from build123d import *

# Parameters (mm, degrees)
SKETCH_1_R          = 25.5
SKETCH_1_R_2        = 15
EXTRUDE_1_DEPTH     = 2
SKETCH_2_R          = 25.5
SKETCH_2_R_2        = 21.5
EXTRUDE_2_DEPTH     = 2
SKETCH_3_R          = 25.5
SKETCH_3_R_2        = 23.5
EXTRUDE_3_DEPTH     = 7
SKETCH_4_W          = 51
SKETCH_4_H          = 80
SKETCH_4_R          = 23.5
EXTRUDE_4_DEPTH     = 8
FILLET_1_R          = 20
SKETCH_5_W          = 51
SKETCH_5_H          = 5
EXTRUDE_5_DEPTH     = 19.7
SKETCH_6_W          = 40
SKETCH_6_H          = 70
EXTRUDE_6_DEPTH     = 3
CUT_EXTRUDE_1_REACH = 65.975
SKETCH_7_R          = 1.25
SKETCH_8_R          = 75
EXTRUDE_7_DEPTH     = 5
SKETCH_9_R          = 22.5
CUT_EXTRUDE_2_DEPTH = 2
CUT_EXTRUDE_3_REACH = 142.425
SKETCH_10_R         = 1.75


with BuildPart() as part:
    # 스케치1 → 보스-돌출1 (new body)
    with BuildSketch(Plane.XY):
        Circle(SKETCH_1_R)
        Circle(SKETCH_1_R_2, mode=Mode.SUBTRACT)
    extrude(amount=EXTRUDE_1_DEPTH)

    # 스케치2 → 보스-돌출2 (add)
    with BuildSketch(Plane.XY.offset(2)):
        Circle(SKETCH_2_R)
        Circle(SKETCH_2_R_2, mode=Mode.SUBTRACT)
    extrude(amount=EXTRUDE_2_DEPTH)

    # 스케치3 → 보스-돌출3 (add)
    with BuildSketch(Plane.XY.offset(4)):
        Circle(SKETCH_3_R)
        Circle(SKETCH_3_R_2, mode=Mode.SUBTRACT)
    extrude(amount=EXTRUDE_3_DEPTH)

    # 스케치4 → 보스-돌출4 (add)
    with BuildSketch(Plane(origin=(0, 0, 0), x_dir=(-1, 0, 0), z_dir=(0, 0, -1))):
        with Locations((0, -10)):
            Rectangle(SKETCH_4_W, SKETCH_4_H)
        with Locations(Location((0, 0, 0), (0, 0, 180))):
            Circle(SKETCH_4_R, mode=Mode.SUBTRACT)
    extrude(amount=-EXTRUDE_4_DEPTH)

    # 필렛1
    fillet_1_edges = [part.edges().sort_by_distance(p)[0] for p in [
        (-25.5, 30, 4),
        (25.5, 30, 4),
    ]]
    fillet(fillet_1_edges, radius=FILLET_1_R)

    # 스케치5 → 보스-돌출5 (add)
    with BuildSketch(Plane(origin=(0, 0, 0), x_dir=(-1, 0, 0), z_dir=(0, 0, -1))):
        Polygon((-20, 20), (-10, 20), (-10, 17), (-17, 17), (-17, 10), (-20, 10), align=None)
        Polygon((20, 20), (10, 20), (10, 17), (17, 17), (17, 10), (20, 10), align=None)
        with Locations((0, -47.5)):
            Rectangle(SKETCH_5_W, SKETCH_5_H)
    extrude(amount=EXTRUDE_5_DEPTH)

    # 스케치6 → 보스-돌출6 (add)
    with BuildSketch(Plane(origin=(0, 0, -19.7), x_dir=(-1, 0, 0), z_dir=(0, 0, -1))):
        with Locations((0, -15)):
            Rectangle(SKETCH_6_W, SKETCH_6_H)
    extrude(amount=-EXTRUDE_6_DEPTH)

    # 스케치7 → 컷-돌출1 (cut, up to next)
    with BuildSketch(Plane(origin=(0, 0, -19.7), x_dir=(-1, 0, 0), z_dir=(0, 0, -1)), mode=Mode.PRIVATE) as cut_extrude_1_sk1:
        with Locations((-5, 13.85)):
            Circle(SKETCH_7_R)
    cut_extrude_1_tool1 = extrude(cut_extrude_1_sk1.sketch, amount=-CUT_EXTRUDE_1_REACH, mode=Mode.PRIVATE) & part.part
    # 스케치7 → 컷-돌출1 (cut, up to next)
    with BuildSketch(Plane(origin=(0, 0, -19.7), x_dir=(-1, 0, 0), z_dir=(0, 0, -1)), mode=Mode.PRIVATE) as cut_extrude_1_sk2:
        with Locations((5, 13.85)):
            Circle(SKETCH_7_R)
    cut_extrude_1_tool2 = extrude(cut_extrude_1_sk2.sketch, amount=-CUT_EXTRUDE_1_REACH, mode=Mode.PRIVATE) & part.part
    # 스케치7 → 컷-돌출1 (cut, up to next)
    with BuildSketch(Plane(origin=(0, 0, -19.7), x_dir=(-1, 0, 0), z_dir=(0, 0, -1)), mode=Mode.PRIVATE) as cut_extrude_1_sk3:
        with Locations((5, -34.75)):
            Circle(SKETCH_7_R)
    cut_extrude_1_tool3 = extrude(cut_extrude_1_sk3.sketch, amount=-CUT_EXTRUDE_1_REACH, mode=Mode.PRIVATE) & part.part
    # 스케치7 → 컷-돌출1 (cut, up to next)
    with BuildSketch(Plane(origin=(0, 0, -19.7), x_dir=(-1, 0, 0), z_dir=(0, 0, -1)), mode=Mode.PRIVATE) as cut_extrude_1_sk4:
        with Locations((-5, -34.75)):
            Circle(SKETCH_7_R)
    cut_extrude_1_tool4 = extrude(cut_extrude_1_sk4.sketch, amount=-CUT_EXTRUDE_1_REACH, mode=Mode.PRIVATE) & part.part
    # 스케치7 → 컷-돌출1 (cut, up to next)
    with BuildSketch(Plane(origin=(0, 0, -19.7), x_dir=(-1, 0, 0), z_dir=(0, 0, -1)), mode=Mode.PRIVATE) as cut_extrude_1_sk5:
        Polygon((-11, -31.5), (-1, -31.5), (-1, -38), (1, -38), (1, -31.5), (11, -31.5), (11, 10.5), (1, 10.5), (1, 17), (-1, 17), (-1, 10.5), (-11, 10.5), align=None)
    cut_extrude_1_tool5 = extrude(cut_extrude_1_sk5.sketch, amount=-CUT_EXTRUDE_1_REACH, mode=Mode.PRIVATE) & part.part
    add(cut_extrude_1_tool1.solids().sort_by_distance((5, 13.85, -19.7))[0], mode=Mode.SUBTRACT)
    add(cut_extrude_1_tool2.solids().sort_by_distance((-5, 13.85, -19.7))[0], mode=Mode.SUBTRACT)
    add(cut_extrude_1_tool3.solids().sort_by_distance((-5, -34.75, -19.7))[0], mode=Mode.SUBTRACT)
    add(cut_extrude_1_tool4.solids().sort_by_distance((5, -34.75, -19.7))[0], mode=Mode.SUBTRACT)
    add(cut_extrude_1_tool5.solids().sort_by_distance((0, -10.5, -19.7))[0], mode=Mode.SUBTRACT)

    # 스케치8 → 보스-돌출7 (add)
    with BuildSketch(Plane.XZ.offset(50)):
        with Locations(Location((0, 14.5, 0), (0, 0, 270))):
            Circle(SKETCH_8_R)
    extrude(amount=-EXTRUDE_7_DEPTH)

    # 스케치9 → 컷-돌출2 (cut)
    with BuildSketch(Plane.XZ.offset(50)):
        with Locations(Location((0, 14.5, 0), (0, 0, 270))):
            Circle(SKETCH_9_R)
    extrude(amount=-CUT_EXTRUDE_2_DEPTH, mode=Mode.SUBTRACT)

    # 스케치10 → 컷-돌출3 (cut, up to next)
    with BuildSketch(Plane.XZ.offset(48), mode=Mode.PRIVATE) as cut_extrude_3_sk1:
        with Locations(Location((0, 33.25, 0), (0, 0, 270))):
            Circle(SKETCH_10_R)
    cut_extrude_3_tool1 = extrude(cut_extrude_3_sk1.sketch, amount=-CUT_EXTRUDE_3_REACH, mode=Mode.PRIVATE) & part.part
    # 스케치10 → 컷-돌출3 (cut, up to next)
    with BuildSketch(Plane.XZ.offset(48), mode=Mode.PRIVATE) as cut_extrude_3_sk2:
        with Locations(Location((13.258252147, 27.758252147, 0), (0, 0, 270))):
            Circle(SKETCH_10_R)
    cut_extrude_3_tool2 = extrude(cut_extrude_3_sk2.sketch, amount=-CUT_EXTRUDE_3_REACH, mode=Mode.PRIVATE) & part.part
    # 스케치10 → 컷-돌출3 (cut, up to next)
    with BuildSketch(Plane.XZ.offset(48), mode=Mode.PRIVATE) as cut_extrude_3_sk3:
        with Locations(Location((18.75, 14.5, 0), (0, 0, 270))):
            Circle(SKETCH_10_R)
    cut_extrude_3_tool3 = extrude(cut_extrude_3_sk3.sketch, amount=-CUT_EXTRUDE_3_REACH, mode=Mode.PRIVATE) & part.part
    # 스케치10 → 컷-돌출3 (cut, up to next)
    with BuildSketch(Plane.XZ.offset(48), mode=Mode.PRIVATE) as cut_extrude_3_sk4:
        with Locations(Location((0, -4.25, 0), (0, 0, 270))):
            Circle(SKETCH_10_R)
    cut_extrude_3_tool4 = extrude(cut_extrude_3_sk4.sketch, amount=-CUT_EXTRUDE_3_REACH, mode=Mode.PRIVATE) & part.part
    # 스케치10 → 컷-돌출3 (cut, up to next)
    with BuildSketch(Plane.XZ.offset(48), mode=Mode.PRIVATE) as cut_extrude_3_sk5:
        with Locations(Location((-18.75, 14.5, 0), (0, 0, 270))):
            Circle(SKETCH_10_R)
    cut_extrude_3_tool5 = extrude(cut_extrude_3_sk5.sketch, amount=-CUT_EXTRUDE_3_REACH, mode=Mode.PRIVATE) & part.part
    # 스케치10 → 컷-돌출3 (cut, up to next)
    with BuildSketch(Plane.XZ.offset(48), mode=Mode.PRIVATE) as cut_extrude_3_sk6:
        with Locations(Location((-13.258252147, 27.758252147, 0), (0, 0, 270))):
            Circle(SKETCH_10_R)
    cut_extrude_3_tool6 = extrude(cut_extrude_3_sk6.sketch, amount=-CUT_EXTRUDE_3_REACH, mode=Mode.PRIVATE) & part.part
    add(cut_extrude_3_tool1.solids().sort_by_distance((0, -48, 33.25))[0], mode=Mode.SUBTRACT)
    add(cut_extrude_3_tool2.solids().sort_by_distance((13.258252, -48, 27.758252))[0], mode=Mode.SUBTRACT)
    add(cut_extrude_3_tool3.solids().sort_by_distance((18.75, -48, 14.5))[0], mode=Mode.SUBTRACT)
    add(cut_extrude_3_tool4.solids().sort_by_distance((0, -48, -4.25))[0], mode=Mode.SUBTRACT)
    add(cut_extrude_3_tool5.solids().sort_by_distance((-18.75, -48, 14.5))[0], mode=Mode.SUBTRACT)
    add(cut_extrude_3_tool6.solids().sort_by_distance((-13.258252, -48, 27.758252))[0], mode=Mode.SUBTRACT)


solid = part.part
Verification items for the finished model (mm, model axes). A direction names the side the tool comes from. Give positions to 0.01 mm unless a question says otherwise; leave off trailing zeros. Loops run counter-clockwise (first coordinate to the right, second up) from the corner with the lowest first, then second, coordinate; pieces in that order, holes last. Notation, with made-up numbers: (-23.5, 17.5) - (-18.5, 17.5) arc R20 ccw to (-18.5, 29.5) - close; hole circle Ø11 at (13, 0). An arc over 180 degrees is marked (long way). Write each question's results on one line, items separated by ' | '.
1) Mould release check, pull along Z, two halves, no side actions. Record for faces 1 (the cylindrical face through (-2.799, 21.317, 2.986)), 2 (the flat face through (4, 15, 2)), 3 (the flat face through (-13, -12, -16.7)): pulls with the +Z half, pulls with the -Z half, needs draft (parallel to the pull), parting line crosses it, or undercut.
Solution:
face 1: needs draft | face 2: pulls with the +Z half | face 3: undercut
2) Sectioned sample at C-C on z = 19. Record the boundary of the cut face in (x, y), plus the area to 3 significant figures.
Solution:
outline: (-74.86, -50) - (-22.05, -50) - (-22.05, -48) - (22.05, -48) - (22.05, -50) - (74.86, -50) - (74.86, -45) - (-74.86, -45) - close | area: 660 mm2
3) Sectioned sample at A-A on y = -42. Record the boundary of the cut face in (x, z).
Solution:
outline: (-25.5, 0) - (25.5, 0) - (25.5, 8) - (-25.5, 8) - close; (-20, -19.7) - (20, -19.7) - (20, -16.7) - (-20, -16.7) - close
4) Depth check by flat-ended pin: P1, Ø3.5, axis at y = 19, z = -9.5, coming from the -X side; P2, Ø6, axis at y = 19, z = 9.5, coming from the +X side; P3, Ø21.5, axis at x = 10.5, y = -8, coming from the +Z side. Enter the tip coordinate at first touch or a pass-through.
Solution:
P1: x = -20 | P2: x = 24.45 | P3: z = 11
5) Sectioned sample at B-B on y = -4. Record the boundary of the cut face in (x, z).
Solution:
outline: (-25.5, 0) - (-14.46, 0) - (-14.46, 2) - (-21.12, 2) - (-21.12, 4) - (-23.16, 4) - (-23.16, 11) - (-25.18, 11) - (-25.18, 8) - (-25.5, 8) - close; (-20, -19.7) - (-11, -19.7) - (-11, -16.7) - (-20, -16.7) - close; (11, -19.7) - (20, -19.7) - (20, -16.7) - (11, -16.7) - close; (14.46, 0) - (25.5, 0) - (25.5, 8) - (25.18, 8) - (25.18, 11) - (23.16, 11) - (23.16, 4) - (21.12, 4) - (21.12, 2) - (14.46, 2) - close
6) Tool access check on faces 4 (the flat face through (-17, 14, -8)), 5 (the flat face through (0, -48, 15)), 6 (the flat face through (25.5, -18, 4)), 7 (the cylindrical face through (22.4, 7.1, 7.5)), 8 (the flat face through (0, 26, 8)). Record the directions out of +Z, -Z, +X, -X, +Y, -Y that give a thin tool (end or side, any length) a straight path to the whole face; none if there is none.
Solution:
face 4: none | face 5: -Y | face 6: +Z, -Z, +X, +Y | face 7: +Z | face 8: +Z, +Y
7) Sectioned sample at D-D on x = 39.5. Record the boundary of the cut face in (y, z).
Solution:
outline: (-50, -49.26) - (-45, -49.26) - (-45, 78.26) - (-50, 78.26) - close
8) Material ranges on L1, parallel to Y at x = -5, z = -18.7; L2, parallel to Z at x = 11.5, y = -41; L3, parallel to Y at x = 0, z = 7, recorded low to high. Write a range as from..to.
Solution:
L1: -50..-36, -33.5..-31.5, 10.5..12.6, 15.1..20 | L2: -19.7..-16.7, 0..8 | L3: -48..-23.5, 23.5..30
